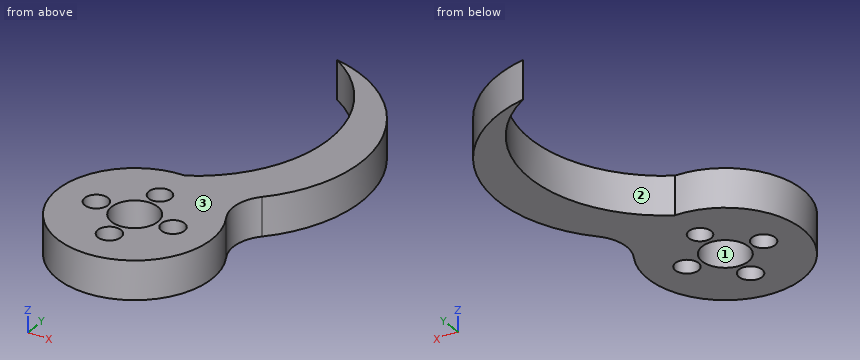
Autodesk Inventor part; units mm, degrees
ref_plane "YZ Plane" through (0, 0, 0) normal (1, 0, 0) x (0, 1, 0)
ref_plane "XZ Plane" through (0, 0, 0) normal (0, 1, 0) x (-1, 0, 0)
ref_plane "XY Plane" through (0, 0, 0) normal (0, 0, 1) x (1, 0, 0)
sketch "Sketch1" plane through (0, 0, 0) normal (0, 0, 1) x (1, 0, 0)
  circle A0 centre (0, 0) radius 12.7
  dimension "d0" = 25.4
extrude "Extrusion1" add sketch "Sketch1" along normal blind 6.35
sketch "Sketch2" plane through (0, 0, 6.35) normal (0, 0, 1) x (1, 0, 0)
  circle A0 centre (0, 0) radius 3.81
  dimension "d3" = 7.62
extrude "Extrusion2" cut sketch "Sketch2" against normal blind 6.35
sketch "Sketch3" plane through (0, 0, 6.35) normal (0, 0, 1) x (1, 0, 0)
  circle A0 centre (0, 6.35) radius 1.8415
  point P0 (0, 0)
  dimension "d6" = 3.683
  dimension "d7" = 6.35
extrude "Extrusion3" cut sketch "Sketch3" against normal blind 6.35
sketch "Sketch4" plane through (0, 0, 6.35) normal (0, 0, 1) x (1, 0, 0)
  circle A0 centre (6.35, 0) radius 1.905
  circle A1 centre (0, -6.35) radius 1.905
  circle A2 centre (-6.35, 0) radius 1.905
  point P0 (0, 0)
  dimension "d10" = 3.81
  dimension "d11" = 3.81
  dimension "d12" = 3.81
  dimension "d13" = 6.35
  dimension "d14" = 6.35
  dimension "d15" = 6.35
extrude "Extrusion4" cut sketch "Sketch4" against normal blind 6.35
sketch "Sketch5" plane through (0, 0, 6.35) normal (0, 0, 1) x (1, 0, 0)
  circle A0 centre (0, 0) radius 12.7
  arc A1 (0, 12.7) -> (0, 50.8) centre (-10.7218, 31.75) ccw
  line L0 (0, 12.7) -> (0, 50.8) construction
  line L1 (0, 12.7) -> (38.1, 12.7) construction
  arc A2 (7.3073, 9.9507) -> (0, 50.8) centre (-3.7987, 29.0422) ccw
  arc A3 (0, 12.7) -> (7.3073, 9.9507) centre (4.4505, 13.4432) ccw
  dimension "d18" = 38.1
  dimension "d19" = 90
extrude "Extrusion5" add sketch "Sketch5" against normal blind 6.35 contours A1 A2 A0 | A0 A2 A3 picked at (3.7894, 11.0049)
fillet "Fillet1" radius 6.35 1 edges at (7.6377, 10.1467, 3.175)
properties part number "claw beta"
Model file for the job. Use its own axes, mm. Face numbers are marked on the shaded views. Coordinates: 2 decimals unless noted, no trailing zeros. Loops run counter-clockwise (first coordinate to the right, second up) from the corner with the lowest first, then second, coordinate; pieces in that order, holes last. Notation, with made-up numbers: M 23,77 L 65,77 A8 ccw 65,81 Z; hole C 25.5,48.5 d4. An arc over 180 degrees is marked long. Use CSV: the item, a comma, the result in double quotes. Start each with the question number.
1. Band-saw the part on B-B, the plane x = -3. List the corners of the cut face in (y, z).
2. Band-saw the part on A-A, the plane y = 0. List the corners of the cut face in (x, z) (3 decimals).
3. Band-saw the part on D-D, the plane z = 5.5. Give the number of separate pieces and of enclosed holes in the cut face, then the cut area to 3 significant figures.
4. Band-saw the part on C-C, the plane x = 6.35. List the corners of the cut face in (y, z) (3 decimals), then the cut area to 3 significant figures.
5. Flat gauge pins, fed straight in: pin 1 (6 mm diameter, centred on x = 0, y = 0, fed in from +Z); pin 2 (2 mm diameter, centred on y = 43.5, z = 3, fed in from -X). Where does each tip first touch, or does it go through?
6. Probe probe 1 along Y at (x, z) = (6.35, 4) (3 decimals); probe 2 along Y at (x, z) = (7, 2.5); probe 3 along X at (y, z) = (1, 0.5). List the from-to ranges inside material, lowest first. Write a range as [from, to].
7. Two-plate mould, pull along Y, no slides. Class the marked faces 1, 2 and 3: pulls with the +Y half, pulls with the -Y half, needs draft (parallel to the pull), parting line crosses it, or undercut.
Entries:
1,outline,"M -12.34,0 L -2.35,0 L -2.35,6.35 L -12.34,6.35 Z; M 2.35,0 L 12.34,0 L 12.34,6.35 L 2.35,6.35 Z"
2,outline,"M -12.7,0 L -8.255,0 L -8.255,6.35 L -12.7,6.35 Z; M -4.445,0 L -3.81,0 L -3.81,6.35 L -4.445,6.35 Z; M 3.81,0 L 4.445,0 L 4.445,6.35 L 3.81,6.35 Z; M 8.255,0 L 12.7,0 L 12.7,6.35 L 8.255,6.35 Z"
3,separate pieces,"1"
3,enclosed holes,"5"
3,area,"695 mm2"
4,outline,"M -10.999,0 L -1.905,0 L -1.905,6.35 L -10.999,6.35 Z; M 1.905,0 L 18.097,0 L 18.097,6.35 L 1.905,6.35 Z; M 45.403,0 L 48.659,0 L 48.659,6.35 L 45.403,6.35 Z"
4,area,"181 mm2"
5,pin 1,"passes through"
5,pin 2,"stops at x = 7.03"
6,probe 1,"y = [-10.999, -1.905], [1.905, 18.097], [45.403, 48.659]"
6,probe 2,"y = [-10.6, -1.79], [1.79, 18.95], [44.55, 48.31]"
6,probe 3,"x = [-12.66, -7.97], [-4.73, -3.68], [3.68, 4.73], [7.97, 12.66]"
7,face 1,"undercut"
7,face 2,"undercut"
7,face 3,"needs draft"
